Here's how the part is built. I have some questions about the finished solid (model axes, mm). Face numbers are marked on the shaded views. A direction names the side the tool comes from. Round coordinates to 2 decimals unless told otherwise and drop trailing zeros. Order: outer loops, then holes, each group sorted by start corner. A loop starts at its lowest first (then second) coordinate and runs counter-clockwise, first axis right, second up. Notation, with made-up numbers: (-19, 34) -> (10, 34) arc R11 ccw to (10, 43) -> close; hole circle Ø8 at (39.25, 61.5). An arc over 180 degrees is marked (long way). One line per item, written item: value.
```python
from build123d import *

# Parameters (mm, degrees)
F0_W     = 12
F0_H     = 12
F1_DEPTH = 3
F2_W     = 12
F2_H     = 6
F3_DEPTH = 10
F4_W     = 12
F4_H     = 3
F4_H_2   = 6
F5_DEPTH = 15


with BuildPart() as f1:
    # F0 (on Top) → F1 (new body)
    with BuildSketch(Plane.XY):
        with Locations((-6, 6)):
            Rectangle(F0_W, F0_H)
    extrude(amount=F1_DEPTH)

    # F2 (on face) → F3 (join)
    with BuildSketch(Plane.XY.offset(3)):
        with Locations((-6, 6)):
            Rectangle(F2_W, F2_H)
    extrude(amount=F3_DEPTH)

    # F4 (on face) → F5 (join)
    with BuildSketch(Plane.XY.offset(13)):
        with Locations((-6, 1.5)):
            Rectangle(F4_W, F4_H)
        with Locations((-6, 6)):
            Rectangle(F4_W, F4_H_2)
        with Locations((-6, 10.5)):
            Rectangle(F4_W, F4_H)
    extrude(amount=F5_DEPTH)


solid = f1.part
```
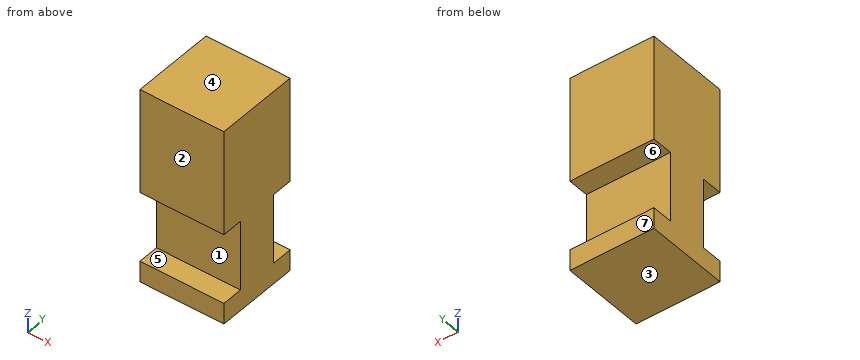
Q1. For P1, Ø3, axis at x = -7.5, z = 6.5, coming from the +Y side; P2, Ø3, axis at x = -4, z = 10.5, coming from the -Y side, each with a flat end and sliding along its axis, tell me the tip position at first contact or that it passes through.
Answers:
P1: y = 9
P2: y = 3
Q2. I want a section at A-A on y = 2.25. Write out the boundary of the cut face in (x, z).
Answers:
outline: (-12, 0) -> (0, 0) -> (0, 3) -> (-12, 3) -> close; (-12, 13) -> (0, 13) -> (0, 28) -> (-12, 28) -> close
Q3. I want a section at C-C on z = 5.75. Write out the boundary of the cut face in (x, y).
Answers:
outline: (-12, 3) -> (0, 3) -> (0, 9) -> (-12, 9) -> close
Q4. I want a section at B-B on x = -9.5. Write out the boundary of the cut face in (y, z), then the cut area to 3 significant figures.
Answers:
outline: (0, 0) -> (12, 0) -> (12, 3) -> (9, 3) -> (9, 13) -> (12, 13) -> (12, 28) -> (0, 28) -> (0, 13) -> (3, 13) -> (3, 3) -> (0, 3) -> close
area: 276 mm2
Q5. Which directions (+Z, -Z, +X, -X, +Y, -Y) give clear straight access to the entire face, cutting with the end or side of a thin tool? Please do the marked faces 5, 6 and 7.
Answers:
face 5: +X, -X, -Y
face 6: +X, -X, +Y
face 7: +Z, -Z, +X, -X, +Y
Q6. If we mould it in two halves opening along Z, with no side actions, what happens to the marked faces 1, 2, 3 and 4? For each: pulls with the +Z half, pulls with the -Z half, needs draft (parallel to the pull), parting line crosses it, or undercut.
Answers:
face 1: undercut
face 2: needs draft
face 3: pulls with the -Z half
face 4: pulls with the +Z half
Q7. I need wall thicknesses on line 1 along Z through (x, y) = (-7, 0.5); line 2 along Y through (x, z) = (-7.5, 3.5). Which ranges of each line are inside material? Lowest first, please.
Answers:
line 1: 0 to 3, 13 to 28
line 2: 3 to 9
